Read the model definition and answer for the solid it produces. Units are mm, in the model's axes. Give positions to 0.01 mm unless a question says otherwise; leave off trailing zeros. Loops run counter-clockwise (first coordinate to the right, second up) from the corner with the lowest first, then second, coordinate; pieces in that order, holes last. Notation, with made-up numbers: (34.5, 23.5) -> (47.5, 23.5) arc R20 ccw to (47.5, 51.5) -> close; hole circle Ø5 at (16.5, 30). An arc over 180 degrees is marked (long way). Write each question's results on one line, items separated by ' | '. Start each with the question number.
Item 1: Section C-C on x = 50 is taken. Write down the section's boundary in (y, z), and give its area (3 significant figures).
Item 2: Section A-A on y = 20 is taken. Write down the section's boundary in (x, z).
Item 3: Section B-B on x = 10 is taken. Write down the section's boundary in (y, z), and give its area (3 significant figures).
Item 4: Each of these flat-tipped pins is pushed along its axis until it touches: P1, Ø5, axis at x = 40, y = -20, coming from the -Z side; P2, Ø8, axis at x = 50, y = 20, coming from the -Z side; P3, Ø7, axis at x = -10, y = -20, coming from the -Z side. Where does it stop, or does it pass through?
Item 5: Find the intervals of material crossed by line 1 (Y direction, x = -10, z = 3.2); line 2 (Y direction, x = 10, z = 3.3); line 3 (X direction, y = 43.5, z = 1.35), in increasing order.
Item 6: Section D-D on y = 40 is taken. Write down the section's boundary in (x, z), and give its area (3 significant figures).
Item 7: Determine the mould class of faces 1 (the cylindrical face through (47, 20.1, 3.2)), 2 (the flat face through (19, 1, 3.416)), 3 (the conical face through (7.504, -41.914, 2.854)) for opening direction Z: +Z half, -Z half, draft (parallel to the pull), parting line (faces both ways), or undercut.
```python
from build123d import *

# Parameters (mm, degrees)
BOSS_EXTRUDE1_DEPTH = 3.416
SKETCH2_R           = 3
CUT_EXTRUDE1_DEPTH  = 4.416
CHAMFER1_SIZE       = 3


with BuildPart() as part:
    # Sketch1 → Boss-Extrude1 (new body)
    with BuildSketch(Plane.XY):
        Polygon((-20, -50), (20, -50), (60, -30), (60, 30), (20, 50), (-20, 50), align=None)
    extrude(amount=BOSS_EXTRUDE1_DEPTH)

    # Sketch2 → Cut-Extrude1 (cut, through all)
    with BuildSketch(Plane.XY.offset(3.416)):
        with Locations((-10, 20)):
            Circle(SKETCH2_R)
        with Locations((10, 40)):
            Circle(SKETCH2_R)
        with Locations((30, 20)):
            Circle(SKETCH2_R)
        with Locations((50, 20)):
            Circle(SKETCH2_R)
        with Locations((-10, -20)):
            Circle(SKETCH2_R)
        with Locations((10, -40)):
            Circle(SKETCH2_R)
        with Locations((40, -20)):
            Circle(SKETCH2_R)
    extrude(amount=-CUT_EXTRUDE1_DEPTH, mode=Mode.SUBTRACT)

    # Chamfer1
    chamfer1_edges = [part.edges().sort_by_distance(p)[0] for p in [
        (-13, -20, 0),
        (47, 20, 0),
        (27, 20, 0),
        (7, 40, 0),
        (7, -40, 0),
        (37, -20, 0),
        (-13, 20, 0),
    ]]
    chamfer(chamfer1_edges, length=CHAMFER1_SIZE)


solid = part.part
```
Findings:
1) outline: (-35, 0) -> (14, 0) -> (17, 3) -> (17, 3.42) -> (-35, 3.42) -> close; (23, 3) -> (26, 0) -> (35, 0) -> (35, 3.42) -> (23, 3.42) -> close | area: 210 mm2
2) outline: (-20, 0) -> (-16, 0) -> (-13, 3) -> (-13, 3.42) -> (-20, 3.42) -> close; (-7, 3) -> (-4, 0) -> (24, 0) -> (27, 3) -> (27, 3.42) -> (-7, 3.42) -> close; (33, 3) -> (36, 0) -> (44, 0) -> (47, 3) -> (47, 3.42) -> (33, 3.42) -> close; (53, 3) -> (56, 0) -> (60, 0) -> (60, 3.42) -> (53, 3.42) -> close
3) outline: (-50, 0) -> (-46, 0) -> (-43, 3) -> (-43, 3.42) -> (-50, 3.42) -> close; (-37, 3) -> (-34, 0) -> (34, 0) -> (37, 3) -> (37, 3.42) -> (-37, 3.42) -> close; (43, 3) -> (46, 0) -> (50, 0) -> (50, 3.42) -> (43, 3.42) -> close | area: 283 mm2
4) P1: through | P2: z = 2 | P3: z = 2.5
5) line 1: -50 to -23, -17 to 17, 23 to 50 | line 2: -50 to -43, -37 to 37, 43 to 50 | line 3: -20 to 6.94, 13.06 to 33
6) outline: (-20, 0) -> (4, 0) -> (7, 3) -> (7, 3.42) -> (-20, 3.42) -> close; (13, 3) -> (16, 0) -> (40, 0) -> (40, 3.42) -> (13, 3.42) -> close | area: 175 mm2
7) face 1: draft | face 2: +Z half | face 3: -Z half
